Could you check a few things on this model? Use its own coordinates, in mm. Face numbers are marked on the shaded views. A direction names the side the tool comes from. Round coordinates to 2 decimals unless told otherwise and drop trailing zeros. Loops run counter-clockwise (first coordinate to the right, second up) from the corner with the lowest first, then second, coordinate; pieces in that order, holes last. Notation, with made-up numbers: (-33.5, -20) - (-9.5, -20) arc R29 cw to (-9.5, 2) - close; hole circle Ø7 at (46, 88.25). An arc over 180 degrees is marked (long way). Use one line per item in the form item = value.
```python
from build123d import *

# Parameters (mm, degrees)
F0_W      = 184.214562
F0_H      = 112.362482
F1_DEPTH  = 101.6
F2_R      = 50.916607
F3_DEPTH  = 19.05
F3_FACE_R = 50.916607
F4_DEPTH  = 149.86
F6_DEPTH  = 330.2
F7_R      = 12.615392
F7_R_2    = 14.70042
F8_DEPTH  = 254
F9_R      = 30.176395
F10_DEPTH = 381


with BuildPart() as f1:
    # F0 (on Top) → F1 (new body)
    with BuildSketch(Plane.XY):
        Rectangle(F0_W, F0_H)
    extrude(amount=F1_DEPTH)

    # F2 (on face) → F3 (join)
    with BuildSketch(Plane.XZ.offset(56.181241)):
        with Locations((0, 101.6)):
            Circle(F2_R)
    extrude(amount=F3_DEPTH)

    # F3_face (on face) → F4 (join)
    with BuildSketch(Plane(origin=(0, -75.231241, 101.6), x_dir=(1, 0, 0), z_dir=(0, -1, 0))):
        Circle(F3_FACE_R)
    extrude(amount=-F4_DEPTH)

    # F5 (on face) → F6 (cut)
    with BuildSketch(Plane.XZ.offset(75.231241)):
        with BuildLine():
            Line((-50.915336, 101.240156), (50.915342, 101.241072))
            ThreePointArc((50.915342, 101.241072), (50.916291, 101.420535), (50.916607, 101.6))
            ThreePointArc((50.916607, 101.6), (-0.179923, 152.51629), (-50.915336, 101.240156))
        make_face()
    extrude(amount=-F6_DEPTH, mode=Mode.SUBTRACT)

    # F7 (on face) → F8 (cut)
    with BuildSketch(Plane.XY.offset(101.6)):
        with Locations((-70.830584, 0)):
            Circle(F7_R)
        with Locations((72.924256, 0)):
            Circle(F7_R_2)
    extrude(amount=-F8_DEPTH, mode=Mode.SUBTRACT)

    # F9 (on face) → F10 (cut)
    with BuildSketch(Plane.XZ.offset(75.231241)):
        with Locations((3e-06, 101.240614)):
            Circle(F9_R)
    extrude(amount=-F10_DEPTH, mode=Mode.SUBTRACT)


solid = f1.part
```
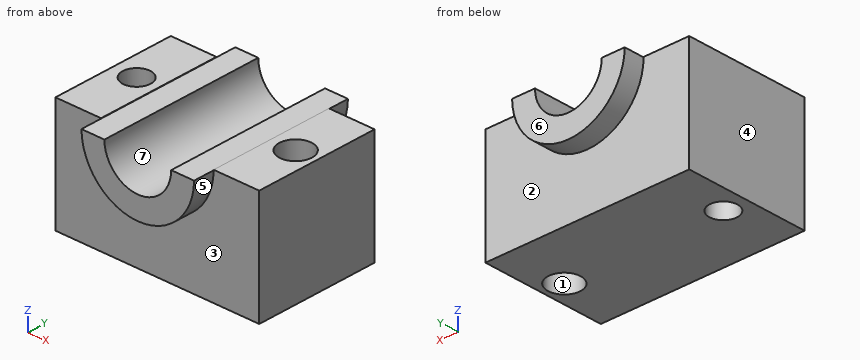
1. If we section it at D-D, the plane y = 32: Write out the boundary of the cut face in (x, z).
Solution:
outline = (-92.11, 0) - (92.11, 0) - (92.11, 101.6) - (50.92, 101.6) arc R50.88 cw to (50.92, 101.24) - (30.18, 101.24) arc R30.18 cw to (-30.18, 101.24) - (-50.92, 101.24) arc R50.92 cw to (-50.92, 101.6) - (-92.11, 101.6) - close
2. If we section it at C-C, the plane x = 0: Write out the boundary of the cut face in (y, z).
Solution:
outline = (-75.23, 50.68) - (-56.18, 50.68) - (-56.18, 0) - (56.18, 0) - (56.18, 50.68) - (74.63, 50.68) - (74.63, 71.06) - (-75.23, 71.06) - close
3. On a 3-axis mill with a long thin cutter (end or side, diameter ignored), from which of +Z, -Z, +X, -X, +Y, -Y can I reach the whole of each face in a straight line? I mean the marked faces 1, 2 and 3. Say none if no direction works.
Solution:
face_1 = +Z, -Z
face_2 = -Z, +Y
face_3 = -Z, -Y
4. We'd pull the mould along X, two halves only. Please class the marked faces 4, 5, 6 and 7: +X half, -X half, draft (parallel to the pull), parting line (faces both ways), or undercut.
Solution:
face_4 = -X half
face_5 = parting line
face_6 = draft
face_7 = undercut
5. If we section it at A-A, the plane y = 0: Write out the boundary of the cut face in (x, z).
Solution:
outline = (-92.11, 0) - (-83.45, 0) - (-83.45, 101.6) - (-92.11, 101.6) - close; (-58.22, 0) - (58.22, 0) - (58.22, 101.6) - (50.92, 101.6) arc R50.88 cw to (50.92, 101.24) - (30.18, 101.24) arc R30.18 cw to (-30.18, 101.24) - (-50.92, 101.24) arc R50.92 cw to (-50.92, 101.6) - (-58.22, 101.6) - close; (87.62, 0) - (92.11, 0) - (92.11, 101.6) - (87.62, 101.6) - close
6. For P1, Ø12, axis at x = -28.5, y = 47.5, coming from the +Z side; P2, Ø3, axis at x = -65, z = 52.5, coming from the -Y side; P3, Ø10, axis at x = -18, y = -15.5, coming from the +Z side, each with a flat end and sliding along its axis, tell me the tip position at first contact or that it passes through.
Solution:
P1 = 101.24
P2 = -56.18
P3 = 81.71
7. Please list where these lines run through material, in increasing order: line 1 along Y through (x, z) = (-51, 59); line 2 along Z through (x, y) = (-41.5, 20); line 3 along Y through (x, z) = (-72, 78.5).
Solution:
line_1 = -56.18 to 56.18
line_2 = 0 to 101.24
line_3 = -56.18 to -12.56, 12.56 to 56.18
8. If we section it at B-B, the plane z = 95: Write out the boundary of the cut face in (x, y), plus the area to 3 significant figures.
Solution:
outline = (-92.11, -56.18) - (-50.49, -56.18) - (-50.49, -75.23) - (-29.52, -75.23) - (-29.52, 74.63) - (-50.49, 74.63) - (-50.49, 56.18) - (-92.11, 56.18) - close; (29.52, -75.23) - (50.49, -75.23) - (50.49, -56.18) - (92.11, -56.18) - (92.11, 56.18) - (50.49, 56.18) - (50.49, 74.63) - (29.52, 74.63) - close; hole circle Ø25.23 at (-70.83, 0); hole circle Ø29.4 at (72.92, 0)
area = 14,500 mm^2
